Check sheet for the modelled part. Datum: model origin and axes. Units: mm. Face numbers are marked on the shaded views. A direction names the side the tool comes from. Give positions to 0.01 mm unless a question says otherwise; leave off trailing zeros. Write each loop counter-clockwise with the first axis right and the second up, starting at its lowest first coordinate (ties: lowest second). Pieces come first, ordered by that corner, then holes. Notation, with made-up numbers: (31.5, -23.5) -> (59.5, -23.5) arc R23 ccw to (59.5, -7.5) -> close; hole circle Ø3 at (-27, -6). An arc over 180 degrees is marked (long way). Answer as a JSON object with one key per item and string values.
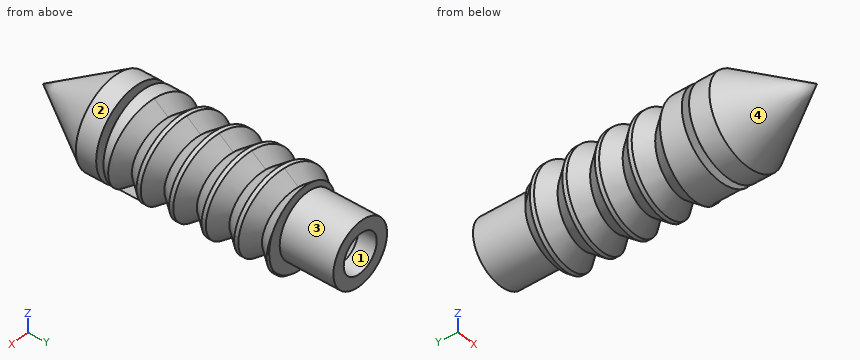
from build123d import *

# Parameters (mm, degrees)
CUT_SWEEP9_PITCH = 1.953846154


with BuildPart() as part:
    # Sketch1 → Revolve1 (revolve)
    with BuildSketch(Plane.XY):
        Polygon((0, 0), (2.697104334, 4.218980763), (2.697104334, 5.438459147), (1.935104334, 5.438459147), (1.935104334, 5.875667474), (2.697104334, 5.875667474), (2.697104334, 15.825259324), (1.935104334, 15.825259324), (1.935104334, 19.05), (1.190625, 19.05), (1.190625, 17.937222993), (0, 15.875), align=None)
    revolve(axis=Axis((0, 0, 0), (0, 1, 0)))

    # Cut-Sweep9: arcs per turn and ends read off the stored shape
    # Cut-Sweep9: the profile of Sketch4 profile screwed along a left-hand helix through 5.4 turns, 10 arcs to a turn; built about Z, then put on its axis
    cut_sweep9_z = Axis((0, 0, 0), (0, 0, 1))
    cut_sweep9_corners = [(2.012993376, -5.973e-06, -1.465383693), (2.697404334, -8.003e-06, -0.615087903), (2.697404334, -8.003e-06, -2.315679482)]
    with BuildLine(mode=Mode.PRIVATE) as cut_sweep9_profile:
        Line(cut_sweep9_corners[0], cut_sweep9_corners[1])
        Line(cut_sweep9_corners[1], cut_sweep9_corners[2])
        Line(cut_sweep9_corners[2], cut_sweep9_corners[0])
    cut_sweep9_cap = Face(cut_sweep9_profile.wire())
    cut_sweep9_turn_angles = [0, -18, -36, -54, -72, -90, -108, -126, -144, -162, -180, -198, -216, -234, -252, -270, -288, -306, -324, -342, -360]
    cut_sweep9_turn_weights = [1, 0.9510565162951535, 1, 0.9510565162951535, 1, 0.9510565162951535, 1, 0.9510565162951535, 1, 0.9510565162951535, 1, 0.9510565162951535, 1, 0.9510565162951535, 1, 0.9510565162951535, 1, 0.9510565162951535, 1, 0.9510565162951535, 1]
    cut_sweep9_turn_rails = [Edge.make_bspline([Vector(p[0], p[1], 0).rotate(cut_sweep9_z, cut_sweep9_turn_angles[k]) / cut_sweep9_turn_weights[k] + Vector(0, 0, p[2] + -CUT_SWEEP9_PITCH * cut_sweep9_turn_angles[k] / 360) for k in range(21)], [0, 0, 0, 1, 1, 2, 2, 3, 3, 4, 4, 5, 5, 6, 6, 7, 7, 8, 8, 9, 9, 10, 10, 10], 2, cut_sweep9_turn_weights) for p in cut_sweep9_corners]
    cut_sweep9_turn_sides = [Face.make_surface_from_curves(cut_sweep9_turn_rails[p[0]], cut_sweep9_turn_rails[p[1]]) for p in [(0, 1), (1, 2), (2, 0)]]
    cut_sweep9_last_angles = [-1800, -1818, -1836, -1854, -1872, -1890, -1908, -1926, -1944]
    cut_sweep9_last_weights = [1, 0.9510565162951535, 1, 0.9510565162951535, 1, 0.9510565162951535, 1, 0.9510565162951382, 1]
    cut_sweep9_last_rails = [Edge.make_bspline([Vector(p[0], p[1], 0).rotate(cut_sweep9_z, cut_sweep9_last_angles[k]) / cut_sweep9_last_weights[k] + Vector(0, 0, p[2] + -CUT_SWEEP9_PITCH * cut_sweep9_last_angles[k] / 360) for k in range(9)], [0, 0, 0, 1, 1, 2, 2, 3, 3, 4, 4, 4], 2, cut_sweep9_last_weights) for p in cut_sweep9_corners]
    cut_sweep9_last_sides = [Face.make_surface_from_curves(cut_sweep9_last_rails[p[0]], cut_sweep9_last_rails[p[1]]) for p in [(0, 1), (1, 2), (2, 0)]]
    cut_sweep9 = Plane(origin=(0, 15.825259324, 0), x_dir=(0, 0, 1), z_dir=(0, -1, 0)) * Solid(Shell([*[p.moved(Location((0, 0, CUT_SWEEP9_PITCH * i))) for i in range(5) for p in cut_sweep9_turn_sides], *cut_sweep9_last_sides, cut_sweep9_cap, cut_sweep9_cap.rotate(cut_sweep9_z, -1944).moved(Location((0, 0, -CUT_SWEEP9_PITCH * -1944 / 360)))]))
    add(cut_sweep9, mode=Mode.SUBTRACT)


solid = part.part
1. Go/stop test with flat-tipped pins: P1, Ø1, axis at x = 2, y = 8, coming from the +Z side; P2, Ø1, axis at y = 12, z = -1.5, coming from the -X side. Record where each tip stops, or that it passes through.
Determined:
{"P1": "z = 2.22", "P2": "x = -2.08"}
2. Access from +Z, -Z, +X, -X, +Y, -Y to the whole of each face (thin tool, end or side, straight path). Record for the marked faces 3 and 4.
Determined:
{"face 3": "+Y", "face 4": "-Y"}
3. Scan lines: L1, parallel to Z at x = 0, y = 18.8; L2, parallel to Y at x = -0.8, z = 1.8. Record each from-to range of solid material in increasing order. Write a range as [from, to].
Determined:
{"L1": "[-1.94, -1.19], [1.19, 1.94]", "L2": "[3.08, 5.44], [5.88, 15.83]"}
4. Sectioned sample at B-B, the plane y = 3. Enter the section's corners in (x, z).
Determined:
{"outline": "circle Ø3.84 at (0, 0)"}
5. Sectioned sample at A-A, the plane y = 16.5. Enter the section's corners in (x, z).
Determined:
{"outline": "circle Ø3.87 at (0, 0); hole circle Ø0.72 at (0, 0)"}
6. Mould release check, pull along Z, two halves, no side actions. Record for the marked faces 1 and 2: released by +Z, released by -Z, zero draft, split by the parting line, or undercut.
Determined:
{"face 1": "undercut", "face 2": "split by the parting line"}
